Work out the finished part from the listing and answer in its coordinate system (mm). A direction names the side the tool comes from. Coordinates: 2 decimals unless noted, no trailing zeros. Loops run counter-clockwise (first coordinate to the right, second up) from the corner with the lowest first, then second, coordinate; pieces in that order, holes last. Notation, with made-up numbers: (15, 62.5) - (73, 62.5) arc R27 ccw to (73, 96.5) - close; hole circle Ø8 at (-26.5, -36.5). An arc over 180 degrees is marked (long way). Write each question's results on one line, items separated by ' | '. Start each with the question number.
1. A cutting plane is placed at A-A on y = 25. Determine the outline of the cut face in (x, z).
2. Each of these flat-tipped pins is pushed along its axis until it touches: P1, Ø0.5, axis at x = -12, z = -2, coming from the +Y side; P2, Ø2, axis at x = -12, z = -2.5, coming from the +Y side; P3, Ø5, axis at x = -10, y = -24, coming from the +Z side; P4, Ø2, axis at x = -12, z = -2.5, coming from the -Y side. Where does it stop, or does it pass through?
3. Find the intervals of material crossed by line 1 along Y through (x, z) = (0, -2.5); line 2 along X through (y, z) = (-1, -1.4); line 3 along Z through (x, y) = (12, 25), in increasing order. Write a range as [from, to].
4. Determine the mould class of faces 4 (the cylindrical face through (-7.5, -26, -2.5)), 5 (the flat face through (6, 29, -2)), 6 (the flat face through (0, 30.5, -2)) for opening direction X: released by +X, released by -X, zero draft, split by the parting line, or undercut.
5. Which of the six approach directions +Z, -Z, +X, -X, +Y, -Y give full straight-line access (tool end or side, diameter ignored) to faces 1 (the flat face through (12.15, 0, -2)), 2 (the cylindrical face through (-11.305, 24.306, -2.138)), 3 (the flat face through (-6, -29, -2))?
6. A cutting plane is placed at B-B on z = -1.15. State how many separate pieces and enclosed holes the cut face has, then the cut area to 3 significant figures.
7. A cutting plane is placed at D-D on x = -6.75. Determine the outline of the cut face in (y, z), then the cut area to 3 significant figures.
8. A cutting plane is placed at C-C on x = 0. Determine the outline of the cut face in (y, z).
Autodesk Inventor part; units mm, degrees
ref_plane "YZ Plane" through (0, 0, 0) normal (1, 0, 0) x (0, 1, 0)
ref_plane "XZ Plane" through (0, 0, 0) normal (0, 1, 0) x (-1, 0, 0)
ref_plane "XY Plane" through (0, 0, 0) normal (0, 0, 1) x (1, 0, 0)
sketch "Sketch1" plane through (0, 0, 0) normal (0, 0, 1) x (1, 0, 0)
  line L0 (15, 27.5) -> (-15, 27.5)
  line L1 (-15, 27.5) -> (-15, -27.5)
  line L2 (-15, -27.5) -> (15, -27.5)
  line L3 (15, -27.5) -> (15, 27.5)
  line L4 (15, 27.5) -> (-15, -27.5) construction
  line L5 (-15, 27.5) -> (15, -27.5) construction
  line L6 (11.25, 17) -> (-11.25, 17) construction
  line L7 (-11.25, 17) -> (-11.25, -17) construction
  line L8 (-11.25, -17) -> (11.25, -17) construction
  line L9 (11.25, -17) -> (11.25, 17) construction
  line L10 (11.25, 17) -> (-11.25, -17) construction
  line L11 (-11.25, 17) -> (11.25, -17) construction
  line L12 (0, 27.5) -> (0, -27.5) construction
  line L13 (15, 0) -> (-15, 0) construction
  line L14 (6, 27.5) -> (6, 30.5)
  line L15 (6, 30.5) -> (-6, 30.5)
  line L16 (-6, 30.5) -> (-6, 27.5)
  arc A0 (-9, 27.5) -> (-6, 27.5) centre (-7.5, 27.5) ccw
  line L17 (6, -27.5) -> (6, -30.5)
  line L18 (6, -30.5) -> (-6, -30.5)
  line L19 (-6, -30.5) -> (-6, -27.5)
  arc A1 (-6, -27.5) -> (-9, -27.5) centre (-7.5, -27.5) ccw
  line L20 (-12, 27.5) -> (-12, 21.5) construction
  line L21 (0, 30.5) -> (0, 27.5) construction
  line L22 (12, 27.5) -> (12, 21.5) construction
  arc A2 (6, 27.5) -> (9, 27.5) centre (7.5, 27.5) ccw
  line L23 (12, -27.5) -> (12, -21.5) construction
  arc A3 (9, -27.5) -> (6, -27.5) centre (7.5, -27.5) ccw
  line L24 (-14.15, -20) -> (14.15, -20) construction
  line L25 (14.15, -20) -> (14.15, 20) construction
  line L26 (14.15, 20) -> (-14.15, 20) construction
  line L27 (-14.15, 20) -> (-14.15, -20) construction
  line L28 (-14.15, -20) -> (14.15, 20) construction
  line L29 (14.15, -20) -> (-14.15, 20) construction
  arc A4 (-12.15, -5.85) -> (12.15, -5.85) centre (0, -5.85) ccw
  line L30 (12.15, -5.85) -> (-12.15, -5.85) construction
  arc A5 (12.15, 5.85) -> (-12.15, 5.85) centre (0, 5.85) ccw
  line L31 (-12.15, -5.85) -> (-12.15, 5.85)
  line L32 (12.15, 5.85) -> (12.15, -5.85)
  circle A6 centre (11.25, 17) radius 1.5 construction
  point P0 (0, 0)
  point P1 (0, 0)
  point P2 (0, 0)
  point P3 (-9, -27.5)
  point P4 (6, -27.5)
  point P5 (-6, -27.5)
  point P6 (-6, -27.5)
  point P7 (6, -27.5)
  point P8 (9, -27.5)
  point P9 (0, 25)
  point P10 (0, -25)
  dimension "d0" = 22.5
  dimension "d1" = 34
  dimension "d19" = 3
  dimension "d37" = 55
  dimension "d40" = 6
  dimension "d41" = 6
  dimension "d57" = 30
  dimension "d58" = 1.5
  dimension "d59" = 28.3
  dimension "d60" = 40
  dimension "d61" = 2
  dimension "d62" = 2
  dimension "d63" = 9
  dimension "d64" = 12
  dimension "d65" = 3
  dimension "d66" = 50
extrude "Extrusion1" add sketch "Sketch1" against normal blind 5 contours L3 L2 A3 A1 L1 L0 A0 A2 | L0 L16 L15 L14 | L17 L18 L19 L2 | L31 A5 L32 A4
extrude "Extrusion2" cut sketch "Sketch1" against normal through all contours L31 A5 L32 A4
hole "M3" at (11.25, 17, 0) at (-11.25, 17, 0) at (-11.25, -17, 0) at (11.25, -17, 0) at (0, -25, 0) at (0, 25, 0) direction (0, 0, -1) diameter 2.459 end through all
sketch "Sketch2" plane through (-15, 27.5, 0) normal (0, 1, 0) x (1, 0, 0)
  line L0 (3, 5) -> (3, 0)
  line L1 (30, 0) -> (0, 0)
  line L2 (27, 5) -> (27, 0)
  line L3 (24, 5) -> (30, 5)
  line L4 (0, 5) -> (6, 5)
  point P0 (15, 0)
  point P1 (6, 0)
  point P2 (3, 2.5)
  point P3 (3, 0)
  point P4 (27, 2.5)
hole "Side-M2" at (-12, 27.5, -2.5) at (12, 27.5, -2.5) direction (0, -1, 0) diameter 1.567 depth 6.3
chamfer "C0.5" distance 0.5 angle 45 4 edges at (6, -30.5, -2.5) (-6, -30.5, -2.5) (6, 30.5, -2.5) (-6, 30.5, -2.5)
mirror "Mirror1" about plane through (0, 0, 0) normal (0, 1, 0) of "Side-M2"
properties part number "HeadSpeakerMountFrame" material "Acetal Resin, Black"
Values:
1) outline: (-15, -5) - (-1.23, -5) - (-1.23, 0) - (-15, 0) - close; (1.23, -5) - (15, -5) - (15, 0) - (1.23, 0) - close; hole circle Ø1.57 at (-12, -2.5); hole circle Ø1.57 at (12, -2.5)
2) P1: y = 21.2 | P2: y = 27.5 | P3: z = 0 | P4: y = -27.5
3) line 1: [-30.5, -26.23], [-23.77, -18], [18, 23.77], [26.23, 30.5] | line 2: [-15, -12.15], [12.15, 15] | line 3: [-5, -3.28], [-1.72, 0]
4) face 4: undercut | face 5: released by +X | face 6: zero draft
5) face 1: +Z, -Z | face 2: +Y | face 3: +Z, -Z, -X, -Y
6) separate pieces: 1 | enclosed holes: 7 | area: 931 mm^2
7) outline: (-26.2, -5) - (-15.95, -5) - (-15.95, 0) - (-26.2, 0) - close; (15.95, -5) - (26.2, -5) - (26.2, 0) - (15.95, 0) - close | area: 102 mm^2
8) outline: (-30.5, -5) - (-26.23, -5) - (-26.23, 0) - (-30.5, 0) - close; (-23.77, -5) - (-18, -5) - (-18, 0) - (-23.77, 0) - close; (18, -5) - (23.77, -5) - (23.77, 0) - (18, 0) - close; (26.23, -5) - (30.5, -5) - (30.5, 0) - (26.23, 0) - close
